Autodesk Fusion 360 part; units mm, degrees
sketch "Sketch1" plane through (0, 0, 0) normal (0, 0, 1) x (1, 0, 0)
  line L0 (0, 0) -> (64.8, 0)
  line L1 (64.8, 0) -> (64.8, -4.8432)
  line L2 (64.8, -4.8432) -> (0, -4.8432)
  line L3 (0, -4.8432) -> (0, 0)
  line L4 (0, -4.8432) -> (-5, -4.8432)
  line L5 (-5, -4.8432) -> (-5, 50.1568)
  line L6 (-5, 50.1568) -> (0, 50.1568)
  line L7 (0, 50.1568) -> (0, -4.8432)
  line L8 (64.8, -4.8432) -> (69.8, -4.8432)
  line L9 (69.8, -4.8432) -> (69.8, 50.1568)
  line L10 (69.8, 50.1568) -> (64.8, 50.1568)
  line L11 (64.8, 50.1568) -> (64.8, -4.8432)
  line L12 (64.8, 42.25) -> (64.8, 39.75)
  circle A0 centre (64.8, 41) radius 1
  circle A1 centre (0, 44) radius 1.25
  dimension "d1" = 64.8
  dimension "d2" = 5
  dimension "d3" = 5
  dimension "d4" = 55
  dimension "d5" = 55
  dimension "d6" = 2.5
  dimension "d7" = 2
  dimension "d8" = 2.5
  dimension "d31" = 44
  dimension "d34" = 41
extrude "Extrude1" add sketch "Sketch1" along normal blind 1
sketch "Sketch2" plane through (0, 0, 1) normal (0, 0, 1) x (-1, 0, 0)
  line L0 (0, 0) -> (0, -42.75)
  arc A0 (0, -42.75) -> (0, -45.25) centre (0, -44) ccw
  line L1 (0, -45.25) -> (0, -50.1568)
  line L2 (0, -50.1568) -> (5, -50.1568)
  line L3 (5, -50.1568) -> (5, 4.8432)
  line L4 (5, 4.8432) -> (-69.8, 4.8432)
  line L5 (-69.8, 4.8432) -> (-69.8, -50.1568)
  line L6 (-69.8, -50.1568) -> (-64.8, -50.1568)
  line L7 (-64.8, -50.1568) -> (-64.8, -42)
  arc A1 (-64.8, -42) -> (-64.8, -40) centre (-64.8, -41) ccw
  line L8 (-64.8, -40) -> (-64.8, 0)
  line L9 (-64.8, 0) -> (0, 0)
  line L10 (5, -50.1568) -> (-2.5, -50.1568)
  line L11 (-2.5, -50.1568) -> (-2.5, -30.1568)
  line L12 (-2.5, -30.1568) -> (5, -30.1568)
  line L13 (5, -30.1568) -> (5, -50.1568)
  line L14 (-69.8, -50.1568) -> (-62.3, -50.1568)
  line L15 (-62.3, -50.1568) -> (-62.3, -30.1568)
  line L16 (-62.3, -30.1568) -> (-69.8, -30.1568)
  line L17 (-69.8, -30.1568) -> (-69.8, -50.1568)
  line L18 (5, 4.8432) -> (-69.8, 4.8432)
  line L19 (-69.8, 4.8432) -> (-69.8, -1.6568)
  line L20 (-69.8, -1.6568) -> (5, -1.6568)
  line L21 (5, -1.6568) -> (5, 4.8432)
  dimension "d11" = 7.5
  dimension "d12" = 20
  dimension "d13" = 7.5
  dimension "d14" = 20
  dimension "d25" = 6.5
extrude "Extrude2" [suppressed]
fillet "Fillet1" [suppressed]
fillet "Fillet2" [suppressed]
fillet "Fillet3" [suppressed]
fillet "Fillet4" [suppressed]
fillet "Fillet5" [suppressed]
mirror "Mirror1" [suppressed]
equation "d1 = 64.3 mm + 0.5 mm"
equation "d2 = d3"
equation "d5 = d4"
equation "d11 = d13"
equation "d14 = d12"
equation "d31 = 42 mm + 2 mm"
equation "d34 = 39 mm + 2 mm"
Could you check a few things on this model? Use its own coordinates, in mm. Give positions to 0.01 mm unless a question says otherwise; leave off trailing zeros. Order: outer loops, then holes, each group sorted by start corner. A loop starts at its lowest first (then second) coordinate and runs counter-clockwise, first axis right, second up.
1. I need wall thicknesses on L1, parallel to X at y = 28, z = 0.7; L2, parallel to X at y = 44, z = 0.15; L3, parallel to Y at x = 37.5, z = 0.35. Which ranges of each line are inside material? Lowest first, please.
Answers below:
L1: x = -5 to 0, 64.8 to 69.8
L2: x = -5 to 1.25, 64.8 to 69.8
L3: y = -4.84 to 0
2. Suppose I cut it at C-C (y = 44). Write out the boundary of the cut face in (x, z), plus the area to 4 significant figures.
Answers below:
outline: (-5, 0) - (1.25, 0) - (1.25, 1) - (-5, 1) - close; (64.8, 0) - (69.8, 0) - (69.8, 1) - (64.8, 1) - close
area: 11.25 mm2
3. For pin 1 (8 mm diameter, centred on x = 17.5, y = 7, fed in from -Z), with a flat end and sliding along its axis, tell me the tip position at first contact or that it passes through.
Answers below:
pin 1: passes through
4. Suppose I cut it at D-D (x = 7.5). Write out the boundary of the cut face in (y, z).
Answers below:
outline: (-4.84, 0) - (0, 0) - (0, 1) - (-4.84, 1) - close
5. Suppose I cut it at B-B (z = 0.4). Write out the boundary of the cut face in (x, y), plus the area to 3 significant figures.
Answers below:
outline: (-5, -4.84) - (69.8, -4.84) - (69.8, 50.16) - (64.8, 50.16) - (64.8, 42) arc R1 ccw to (64.8, 40) - (64.8, 0) - (0, 0) - (0, 42.75) arc R1.25 ccw to (0, 45.25) - (0, 50.16) - (-5, 50.16) - close
area: 868 mm2
6. Suppose I cut it at A-A (y = 36). Write out the boundary of the cut face in (x, z).
Answers below:
outline: (-5, 0) - (0, 0) - (0, 1) - (-5, 1) - close; (64.8, 0) - (69.8, 0) - (69.8, 1) - (64.8, 1) - close
